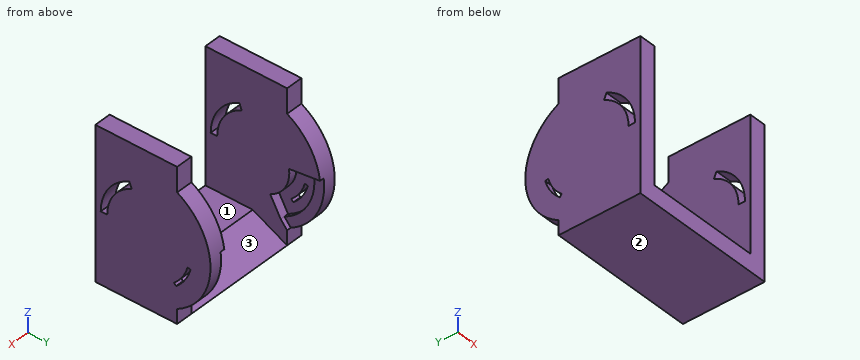
```python
from build123d import *

# Parameters (mm, degrees)
CROQUIS1_W              = 34
CROQUIS1_H              = 19
SALIENTE_EXTRUIR1_DEPTH = 35
CROQUIS2_W              = 26.2
CROQUIS2_H              = 31
CORTAR_EXTRUIR1_DEPTH   = 25
CORTAR_EXTRUIR3_DEPTH   = 26.2
SALIENTE_EXTRUIR2_DEPTH = 34
CROQUIS10_W             = 26.2
CROQUIS10_H             = 25.966324345
CORTAR_EXTRUIR4_DEPTH   = 10
CORTAR_EXTRUIR5_START   = -34
CORTAR_EXTRUIR5_DEPTH   = 34
CORTAR_EXTRUIR6_DEPTH   = 2
CORTAR_EXTRUIR7_START   = 28.2
CORTAR_EXTRUIR7_DEPTH   = 28.2
CORTAR_EXTRUIR8_DEPTH   = 1
CORTAR_EXTRUIR9_DEPTH   = 27.2


with BuildPart() as part:
    # Croquis1 → Saliente-Extruir1 (new body)
    with BuildSketch(Plane.XY):
        with Locations((-31.887263086, 5.12254902)):
            Rectangle(CROQUIS1_W, CROQUIS1_H)
    extrude(amount=SALIENTE_EXTRUIR1_DEPTH)

    # Croquis2 → Cortar-Extruir1 (cut)
    with BuildSketch(Plane.XZ.offset(4.37745098)):
        with Locations((-31.887263086, 19.5)):
            Rectangle(CROQUIS2_W, CROQUIS2_H)
    extrude(amount=-CORTAR_EXTRUIR1_DEPTH, mode=Mode.SUBTRACT)

    # Croquis4 → Cortar-Extruir3 (cut)
    with BuildSketch(Plane.ZY.offset(18.787263086)):
        Polygon((4, 14.62254902), (4, 6.62254902), (0, 14.62254902), align=None)
    extrude(amount=CORTAR_EXTRUIR3_DEPTH, mode=Mode.SUBTRACT)

    # Croquis9 → Saliente-Extruir2 (add)
    with BuildSketch(Plane(origin=(-14.887263086, 0, 0), x_dir=(0, 0, -1), z_dir=(1, 0, 0))):
        with BuildLine():
            Line((-29.315831827, 14.62254902), (-3.349507482, 14.62254902))
            ThreePointArc((-3.349507482, 14.62254902), (-16.332669655, 22.37254902), (-29.315831827, 14.62254902))
        make_face()
    extrude(amount=-SALIENTE_EXTRUIR2_DEPTH)

    # Croquis10 → Cortar-Extruir4 (cut)
    with BuildSketch(Plane.XZ.offset(-14.62254902)):
        with Locations((-31.887263086, 16.332669655)):
            Rectangle(CROQUIS10_W, CROQUIS10_H)
    extrude(amount=-CORTAR_EXTRUIR4_DEPTH, mode=Mode.SUBTRACT)

    # Croquis11 → Cortar-Extruir5 (cut)
    with BuildSketch(Plane(origin=(-14.887263086, 0, 0), x_dir=(0, 0, -1), z_dir=(1, 0, 0)).offset(CORTAR_EXTRUIR5_START)):
        with BuildLine():
            Line((-26.264575199, 3.509186373), (-24.878727914, 4.083143951))
            ThreePointArc((-24.878727914, 4.083143951), (-21.471881808, -0.068419609), (-16.332669655, -1.62745098))
            Line((-16.332669655, -1.62745098), (-16.332669655, -3.12745098))
            ThreePointArc((-16.332669655, -3.12745098), (-22.305267563, -1.31560371), (-26.264575199, 3.509186373))
        make_face()
        with BuildLine():
            Line((-13.621540157, 17.74062205), (-13.807242822, 17.04757027))
            ThreePointArc((-13.807242822, 17.04757027), (-11.089968726, 15.851941052), (-8.857991001, 13.894549121))
            Line((-8.857991001, 13.894549121), (-8.308354113, 14.355749231))
            ThreePointArc((-8.308354113, 14.355749231), (-10.704456257, 16.457074414), (-13.621540157, 17.74062205))
        make_face()
    extrude(amount=CORTAR_EXTRUIR5_DEPTH, mode=Mode.SUBTRACT)

    # Croquis12 → Cortar-Extruir6 (cut)
    with BuildSketch(Plane.ZY.offset(18.787263086)):
        with BuildLine():
            Line((17.258889566, 15.065137056), (17.873210354, 20.027255157))
            ThreePointArc((17.873210354, 20.027255157), (10.39091869, 18.620075808), (5.112868034, 13.133089064))
            Line((5.112868034, 13.133089064), (9.488064371, 10.688715764))
            ThreePointArc((9.488064371, 10.688715764), (12.652304566, 14.157448622), (17.258889566, 15.065137056))
        make_face()
    extrude(amount=-CORTAR_EXTRUIR6_DEPTH, mode=Mode.SUBTRACT)

    # Croquis14 → Cortar-Extruir7 (cut)
    with BuildSketch(Plane.ZY.offset(18.787263086).offset(CORTAR_EXTRUIR7_START)):
        with BuildLine():
            Line((17.873210354, 20.027255157), (17.258889566, 15.065137056))
            ThreePointArc((17.258889566, 15.065137056), (12.652304566, 14.157448622), (9.488064371, 10.688715764))
            Line((9.488064371, 10.688715764), (5.112868034, 13.133089064))
            ThreePointArc((5.112868034, 13.133089064), (10.39091869, 18.620075808), (17.873210354, 20.027255157))
        make_face()
    extrude(amount=-CORTAR_EXTRUIR7_DEPTH, mode=Mode.SUBTRACT)

    # Croquis15 → Cortar-Extruir8 (cut)
    with BuildSketch(Plane.ZY.offset(18.787263086)):
        with BuildLine():
            Line((17.873210354, 20.027255157), (18.15050768, 22.260102262))
            ThreePointArc((18.15050768, 22.260102262), (9.568856329, 20.730307382), (3.349507482, 14.62254902))
            Line((3.349507482, 14.62254902), (5.112868034, 13.133089064))
            ThreePointArc((5.112868034, 13.133089064), (10.39091869, 18.620075808), (17.873210354, 20.027255157))
        make_face()
    extrude(amount=-CORTAR_EXTRUIR8_DEPTH, mode=Mode.SUBTRACT)

    # Croquis15<2> → Cortar-Extruir9 (cut)
    with BuildSketch(Plane.ZY.offset(18.787263086)):
        with BuildLine():
            Line((17.873210354, 20.027255157), (18.15050768, 22.260102262))
            ThreePointArc((18.15050768, 22.260102262), (9.568856329, 20.730307382), (3.349507482, 14.62254902))
            Line((3.349507482, 14.62254902), (5.112868034, 13.133089064))
            ThreePointArc((5.112868034, 13.133089064), (10.39091869, 18.620075808), (17.873210354, 20.027255157))
        make_face()
    extrude(amount=CORTAR_EXTRUIR9_DEPTH, mode=Mode.SUBTRACT)


solid = part.part
```
Check sheet for the modelled part. Datum: model origin and axes. Units: mm. Face numbers are marked on the shaded views. A direction names the side the tool comes from. Round coordinates to 2 decimals unless told otherwise and drop trailing zeros. Loops run counter-clockwise (first coordinate to the right, second up) from the corner with the lowest first, then second, coordinate; pieces in that order, holes last. Notation, with made-up numbers: (-30, 85.25) - (9, 85.25) arc R17 cw to (9, 94.25) - close; hole circle Ø1 at (-9, 65.25). An arc over 180 degrees is marked (long way). Write item = value, one per line. Start each with the question number.
Q1. Section check A-A (y = 1.75). Record the boundary of the cut face in (x, z).
Q2. Depth check by flat-ended pin: P1, Ø1.2, axis at x = -47, z = 33.5, coming from the +Y side; P2, Ø3.5, axis at x = -36, y = 2.5, coming from the +Z side. Enter the tip coordinate at first touch or a pass-through.
Q3. Section check C-C (y = 9.25). Record the boundary of the cut face in (x, z), plus the area to 3 significant figures.
Q4. Access from +Z, -Z, +X, -X, +Y, -Y to the whole of each face (thin tool, end or side, straight path). Record for the marked faces 1, 2 and 3.
Q5. Section check D-D (x = -35). Record the boundary of the cut face in (y, z), plus the area to 3 significant figures.
Q6. Section check B-B (z = 28). Record the boundary of the cut face in (x, y).
Q7. Thickness scan on L1, parallel to X at y = -2, z = 30.5; L2, parallel to X at y = 17.5, z = 14; L3, parallel to Z at x = -45.5, y = 13.5. Record the ranges inside material, lowest first.
Derived:
q1.outline = (-48.89, 0) - (-14.89, 0) - (-14.89, 23.48) - (-18.79, 23.48) - (-18.79, 4) - (-44.99, 4) - (-44.99, 23.48) - (-48.89, 23.48) - close; (-48.89, 25.34) - (-44.99, 25.34) - (-44.99, 35) - (-48.89, 35) - close; (-18.79, 25.34) - (-14.89, 25.34) - (-14.89, 35) - (-18.79, 35) - close
q2.P1 = 14.62
q2.P2 = 4
q3.outline = (-48.89, 0) - (-14.89, 0) - (-14.89, 35) - (-18.79, 35) - (-18.79, 2.69) - (-44.99, 2.69) - (-44.99, 35) - (-48.89, 35) - close
q3.area = 343 mm^2
q4.face_1 = +Z, +Y, -Y
q4.face_2 = -Z, +X, -X, +Y, -Y
q4.face_3 = +Z, +Y
q5.outline = (-4.38, 0) - (14.62, 0) - (6.62, 4) - (-4.38, 4) - close
q5.area = 60.0 mm^2
q6.outline = (-48.89, -4.38) - (-44.99, -4.38) - (-44.99, 16.65) - (-48.89, 16.65) - close; (-18.79, -4.38) - (-14.89, -4.38) - (-14.89, 16.65) - (-18.79, 16.65) - close
q7.L1 = -48.89 to -44.99, -18.79 to -14.89
q7.L2 = -48.89 to -46.99, -16.79 to -14.89
q7.L3 = 0 to 4.68, 11.67 to 35
